```python
from build123d import *

# Parameters (mm, degrees)
F0_R     = 9.5
F1_DEPTH = 5
F3_DEPTH = 25


with BuildPart() as f1:
    # F0 (on Front) → F1 (new body, symmetric)
    with BuildSketch(Plane.XZ):
        with BuildLine():
            ThreePointArc((-15.047428, 68.438281), (-2.760539, 47.239942), (16, 63))
            ThreePointArc((16, 63), (15.760058, 65.760539), (15.047428, 68.438281))
            ThreePointArc((15.047428, 68.438281), (0, 79), (-15.047428, 68.438281))
        make_face()
        with Locations((0, 63)):
            Circle(F0_R, mode=Mode.SUBTRACT)
        with BuildLine():
            ThreePointArc((15.047428, 68.438281), (15.760058, 65.760539), (16, 63))
            ThreePointArc((16, 63), (-2.760539, 47.239942), (-15.047428, 68.438281))
            ThreePointArc((-15.047428, 68.438281), (-32.681379, 44.98206), (-60.438762, 35.459547))
            ThreePointArc((-60.438762, 35.459547), (-48.78901, 30.964923), (-43.916561, 19.468071))
            ThreePointArc((-43.916561, 19.468071), (-52.886354, 5.095312), (-69.738584, 6.837637))
            ThreePointArc((-69.738584, 6.837637), (-52.879582, -17.181618), (-52.400638, -46.523076))
            ThreePointArc((-52.400638, -46.523076), (-34.785773, -35.126311), (-21.030471, -50.968071))
            ThreePointArc((-21.030471, -50.968071), (-22.894818, -58.463625), (-28.053387, -64.212389))
            ThreePointArc((-28.053387, -64.212389), (0, -55.600883), (28.053387, -64.212389))
            ThreePointArc((28.053387, -64.212389), (27.625907, -38.023799), (52.400638, -46.523076))
            ThreePointArc((52.400638, -46.523076), (52.879582, -17.181618), (69.738584, 6.837637))
            ThreePointArc((69.738584, 6.837637), (44.699656, 14.523799), (60.438762, 35.459547))
            ThreePointArc((60.438762, 35.459547), (32.681379, 44.98206), (15.047428, 68.438281))
        make_face()
        with BuildLine():
            ThreePointArc((75.916561, 19.468071), (71.413413, 30.595621), (60.438762, 35.459547))
            ThreePointArc((60.438762, 35.459547), (44.699656, 14.523799), (69.738584, 6.837637))
            ThreePointArc((69.738584, 6.837637), (74.289319, 12.437864), (75.916561, 19.468071))
        make_face()
        with Locations((59.916561, 19.468071)):
            Circle(F0_R, mode=Mode.SUBTRACT)
        with BuildLine():
            ThreePointArc((-43.916561, 19.468071), (-48.78901, 30.964923), (-60.438762, 35.459547))
            ThreePointArc((-60.438762, 35.459547), (-75.133465, 24.412343), (-69.738584, 6.837637))
            ThreePointArc((-69.738584, 6.837637), (-52.886354, 5.095312), (-43.916561, 19.468071))
        make_face()
        with Locations((-59.916561, 19.468071)):
            Circle(F0_R, mode=Mode.SUBTRACT)
        with BuildLine():
            ThreePointArc((53.030471, -50.968071), (52.87223, -48.723373), (52.400638, -46.523076))
            ThreePointArc((52.400638, -46.523076), (27.625907, -38.023799), (28.053387, -64.212389))
            ThreePointArc((28.053387, -64.212389), (44.526025, -65.103723), (53.030471, -50.968071))
        make_face()
        with Locations((37.030471, -50.968071)):
            Circle(F0_R, mode=Mode.SUBTRACT)
        with BuildLine():
            ThreePointArc((-21.030471, -50.968071), (-34.785773, -35.126311), (-52.400638, -46.523076))
            ThreePointArc((-52.400638, -46.523076), (-46.435035, -63.912343), (-28.053387, -64.212389))
            ThreePointArc((-28.053387, -64.212389), (-22.894818, -58.463625), (-21.030471, -50.968071))
        make_face()
        with Locations((-37.030471, -50.968071)):
            Circle(F0_R, mode=Mode.SUBTRACT)
    extrude(amount=F1_DEPTH, both=True)

    # F2 (on face) → F3 (cut)
    with BuildSketch(Plane.XZ.offset(5)):
        with BuildLine():
            Line((21.483138, 12.785725), (26.554308, 17.856895))
            ThreePointArc((26.554308, 17.856895), (22.627417, 22.627417), (17.856895, 26.554308))
            Line((17.856895, 26.554308), (12.785725, 21.483138))
            ThreePointArc((12.785725, 21.483138), (9.567086, 23.096988), (6.15, 24.231746))
            Line((6.15, 24.231746), (6.15, 31.403463))
            ThreePointArc((6.15, 31.403463), (0, 32), (-6.15, 31.403463))
            Line((-6.15, 31.403463), (-6.15, 24.231746))
            ThreePointArc((-6.15, 24.231746), (-9.567086, 23.096988), (-12.785725, 21.483138))
            Line((-12.785725, 21.483138), (-17.856895, 26.554308))
            ThreePointArc((-17.856895, 26.554308), (-22.627417, 22.627417), (-26.554308, 17.856895))
            Line((-26.554308, 17.856895), (-21.483138, 12.785725))
            ThreePointArc((-21.483138, 12.785725), (-23.096988, 9.567086), (-24.231746, 6.15))
            Line((-24.231746, 6.15), (-31.403463, 6.15))
            ThreePointArc((-31.403463, 6.15), (-32, 0), (-31.403463, -6.15))
            Line((-31.403463, -6.15), (-24.231746, -6.15))
            ThreePointArc((-24.231746, -6.15), (-23.096988, -9.567086), (-21.483138, -12.785725))
            Line((-21.483138, -12.785725), (-26.554308, -17.856895))
            ThreePointArc((-26.554308, -17.856895), (-22.627417, -22.627417), (-17.856895, -26.554308))
            Line((-17.856895, -26.554308), (-12.785725, -21.483138))
            ThreePointArc((-12.785725, -21.483138), (-9.567086, -23.096988), (-6.15, -24.231746))
            Line((-6.15, -24.231746), (-6.15, -31.403463))
            ThreePointArc((-6.15, -31.403463), (0, -32), (6.15, -31.403463))
            Line((6.15, -31.403463), (6.15, -24.231746))
            ThreePointArc((6.15, -24.231746), (9.567086, -23.096988), (12.785725, -21.483138))
            Line((12.785725, -21.483138), (17.856895, -26.554308))
            ThreePointArc((17.856895, -26.554308), (22.627417, -22.627417), (26.554308, -17.856895))
            Line((26.554308, -17.856895), (21.483138, -12.785725))
            ThreePointArc((21.483138, -12.785725), (23.096988, -9.567086), (24.231746, -6.15))
            Line((24.231746, -6.15), (31.403463, -6.15))
            ThreePointArc((31.403463, -6.15), (32, 0), (31.403463, 6.15))
            Line((31.403463, 6.15), (24.231746, 6.15))
            ThreePointArc((24.231746, 6.15), (23.096988, 9.567086), (21.483138, 12.785725))
        make_face()
    extrude(amount=-F3_DEPTH, mode=Mode.SUBTRACT)


solid = f1.part
```
CAD build for the part. Positions are in the model's coordinates, mm. A direction names the side the tool comes from. Give positions to 0.01 mm unless a question says otherwise; leave off trailing zeros. Write each loop counter-clockwise with the first axis right and the second up, starting at its lowest first coordinate (ties: lowest second). Pieces come first, ordered by that corner, then holes. Notation, with made-up numbers: (-13.5, 37) -> (-7.5, 37) arc R22 ccw to (-7.5, 67) -> close; hole circle Ø4 at (-20, -37.75). An arc over 180 degrees is marked (long way). Write each question's results on one line, items separated by ' | '.
1. Which spindle directions (+Z, -Z, +X, -X, +Y, -Y) get a long thin tool onto all of the face, cutting with end or side? Do faces 4 (the cylindrical face through (23.08, -0.07, -9.61)), 5 (the cylindrical face through (-53.01, -0.07, -16.79)). Say none if no direction does.
Geometry check:
face 4: +Y, -Y | face 5: -X, +Y, -Y
2. Cut at C-C, the plane x = 36. Write the cut outline in (y, z).
Geometry check:
outline: (-5, -66.93) -> (5, -66.93) -> (5, -60.41) -> (-5, -60.41) -> close; (-5, -41.52) -> (5, -41.52) -> (5, 42.77) -> (-5, 42.77) -> close
3. Wall check: probe 1 along X at (y, z) = (-3.75, -51); probe 2 along Z at (x, y) = (-28.5, 3.75); probe 3 along X at (y, z) = (-4, -29). Give the ranges that are in metal, low to high. Write a range as [from, to].
Geometry check:
probe 1: [-53.03, -46.53], [-27.53, 27.53], [46.53, 53.03] | probe 2: [-64.5, -55.15], [-46.79, -6.15], [6.15, 48.38] | probe 3: [-50.56, -6.15], [6.15, 50.56]
4. Two-plate mould, pull along Z, no slides. Class faces 1 (the cylindrical face through (-75.047, -0.07, 24.672)), 2 (the flat face through (-15.3, -0.1, 24)), 3 (the cylindrical face through (-0.417, -0.07, -55.603)): pulls with the +Z half, pulls with the -Z half, needs draft (parallel to the pull), parting line crosses it, or undercut.
Geometry check:
face 1: parting line crosses it | face 2: undercut | face 3: pulls with the -Z half
5. Cut at B-B, the plane z = 63. Write the cut outline in (x, y).
Geometry check:
outline: (-17.39, -5) -> (-9.5, -5) -> (-9.5, 5) -> (-17.39, 5) -> close; (9.5, -5) -> (17.39, -5) -> (17.39, 5) -> (9.5, 5) -> close
6. Drop flat-ended pins along their axis: P1, Ø5.5, axis at y = -2, z = -29.5, coming from the -X side; P2, Ø5.5, axis at y = -0.5, z = -27, coming from the +X side; P3, Ø2, axis at y = -1, z = 26.5, coming from the -X side. Give the stop position or say it passes through.
Geometry check:
P1: x = -50.78 | P2: x = 51.14 | P3: x = -74.74
7. Cut at D-D, the plane z = -44. Write the cut outline in (x, y), then the cut area to 3 significant figures.
Geometry check:
outline: (-51.74, -5) -> (-43.49, -5) -> (-43.49, 5) -> (-51.74, 5) -> close; (-30.57, -5) -> (30.57, -5) -> (30.57, 5) -> (-30.57, 5) -> close; (43.49, -5) -> (51.74, -5) -> (51.74, 5) -> (43.49, 5) -> close | area: 777 mm²
8. Cut at A-A, the plane x = 0. Write the cut outline in (y, z).
Geometry check:
outline: (-5, -55.6) -> (5, -55.6) -> (5, -32) -> (-5, -32) -> close; (-5, 32) -> (5, 32) -> (5, 53.5) -> (-5, 53.5) -> close; (-5, 72.5) -> (5, 72.5) -> (5, 79) -> (-5, 79) -> close
